Input: part model. Units: mm. Frame: model coordinates. Face numbers are marked on the shaded views. A direction names the side the tool comes from. Coordinates: 2 decimals unless noted, no trailing zeros. Loops run counter-clockwise (first coordinate to the right, second up) from the corner with the lowest first, then second, coordinate; pieces in that order, holes last. Notation, with made-up numbers: (0.5, 70) -> (35.5, 70) arc R24 cw to (35.5, 98) -> close; hole circle Ø9 at (23.25, 32.5). An arc over 180 degrees is marked (long way). Put each result on its own line as item: value. Start each with the question number.
1) Material intervals for L1, parallel to X at y = 1.75, z = -7.25; L2, parallel to Z at x = 7.62, y = 2 (3 decimals); L3, parallel to X at y = 3.25, z = 0.25, sorted ascending.
2) Cut plane B-B (z = -7). Return the cut outline in (x, y), plus the area to 3 significant figures.
3) Set-up query: the marked faces 4, 5, 6, 7 and 8. Return all of +Z, -Z, +X, -X, +Y, -Y with unobstructed straight access to the full face (end or side cutting, diameter ignored); none if empty.
4) Contact query for flat-ended pins moving along their axis: P1, Ø10, axis at x = 3, z = -1.5, coming from the -Y side; P2, Ø1.5, axis at x = 3, z = 2.5, coming from the +Y side; P3, Ø4, axis at x = 0.5, y = -3.5, coming from the -Z side. Output: stop coordinate, or through.
5) Cut plane C-C (x = 4). Return the cut outline in (y, z).
6) Pull-direction query (X, two-part tool) for the marked faces 1, 2 and 3; classes: pulls with the +X half, pulls with the -X half, needs draft (parallel to the pull), parting line crosses it, or undercut.
7) Cut plane D-D (y = -6.75). Return the cut outline in (x, z), plus the area to 3 significant figures.
8) Cut plane A-A (x = 7.62). Return the cut outline in (y, z) (3 decimals).
from build123d import *

# Parameters (mm, degrees)
ESQUISSE1_W        = 20.32
ESQUISSE1_H        = 20.32
BOSS_EXTRU_1_DEPTH = 2.7
D_GAGEMENT_M2_51_D = 2.9
ESQUISSE7_W        = 2
ESQUISSE7_H        = 2.3
ESQUISSE7_W_2      = 1.6
ESQUISSE7_H_2      = 3.2
BOSS_EXTRU_3_DEPTH = 1.1
ESQUISSE3_W        = 18.3
ESQUISSE3_H        = 2.4
BOSS_EXTRU_2_DEPTH = 8.5
CONG_1_R           = 2


with BuildPart() as part:
    # Esquisse1 → Boss.-Extru.1 (new body)
    with BuildSketch(Plane(origin=(0, 0, 0), x_dir=(1, 0, 0), z_dir=(0, 1, 0))):
        Rectangle(ESQUISSE1_W, ESQUISSE1_H)
    extrude(amount=BOSS_EXTRU_1_DEPTH)

    # Dégagement M2.51 (through all)
    with Locations(Plane(origin=(0, 2.7, 0), x_dir=(1, 0, 0), z_dir=(0, 1, 0))):
        with Locations((-7.62, 7.835000674), (7.62, 7.835000674)):
            Hole(D_GAGEMENT_M2_51_D / 2)

    # Esquisse7 → Boss.-Extru.3 (add)
    with BuildSketch(Plane(origin=(0, 2.7, 0), x_dir=(1, 0, 0), z_dir=(0, 1, 0))):
        with Locations((0.254, -0.254)):
            Rectangle(ESQUISSE7_W, ESQUISSE7_H)
        with Locations((-3.048, -0.034)):
            Rectangle(ESQUISSE7_W_2, ESQUISSE7_H_2)
    extrude(amount=BOSS_EXTRU_3_DEPTH)

    # Esquisse3 → Boss.-Extru.2 (add)
    with BuildSketch(Plane(origin=(0, 0, 0), x_dir=(1, 0, 0), z_dir=(0, 1, 0))):
        with Locations((0, -8.636)):
            Rectangle(ESQUISSE3_W, ESQUISSE3_H)
    extrude(amount=-BOSS_EXTRU_2_DEPTH)

    # Congé1
    cong_1_edges = [part.edges().sort_by_distance(p)[0] for p in [
        (-10.16, 1.35, -10.16),
        (10.16, 1.35, -10.16),
        (10.16, 1.35, 10.16),
        (-10.16, 1.35, 10.16),
    ]]
    fillet(cong_1_edges, radius=CONG_1_R)


solid = part.part
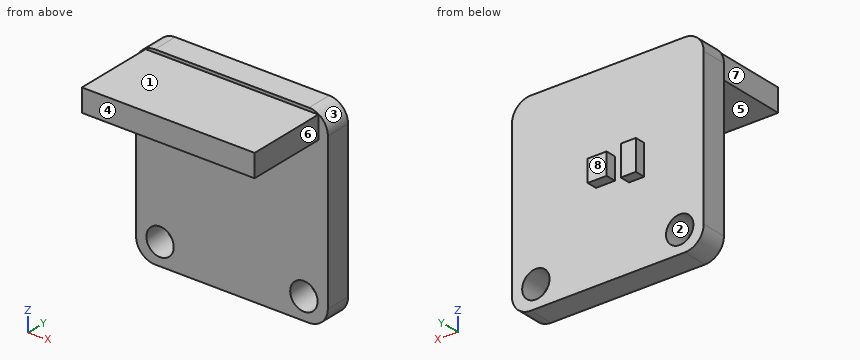
Results found:
1. L1: x = -10.16 to -8.95, -6.29 to 6.29, 8.95 to 10.16
1. L2: z = -10.16 to -9.285, -6.385 to 10.16
1. L3: x = -3.85 to -2.25, -0.75 to 1.25
2. outline: (-10.16, 0) -> (-8.81, 0) -> (-8.81, 2.7) -> (-10.16, 2.7) -> close; (-6.43, 0) -> (6.43, 0) -> (6.43, 2.7) -> (-6.43, 2.7) -> close; (8.81, 0) -> (10.16, 0) -> (10.16, 2.7) -> (8.81, 2.7) -> close
2. area: 42.1 mm2
3. face 4: +Z, -Z, +X, -X, -Y
3. face 5: -Z, +X, -X, -Y
3. face 6: +Z, -Z, +X, -Y
3. face 7: +Z, -Z, -X, -Y
3. face 8: +Z, -Z, +X, -X, +Y
4. P1: stops at y = 0
4. P2: stops at y = 2.7
4. P3: stops at z = 7.44
5. outline: (-8.5, 7.44) -> (0, 7.44) -> (0, -10.16) -> (2.7, -10.16) -> (2.7, 10.16) -> (0, 10.16) -> (0, 9.84) -> (-8.5, 9.84) -> close
6. face 1: needs draft
6. face 2: undercut
6. face 3: pulls with the +X half
7. outline: (-9.15, 7.44) -> (9.15, 7.44) -> (9.15, 9.84) -> (-9.15, 9.84) -> close
7. area: 43.9 mm2
8. outline: (-8.5, 7.436) -> (0, 7.436) -> (0, -6.385) -> (2.7, -6.385) -> (2.7, 10.16) -> (0, 10.16) -> (0, 9.836) -> (-8.5, 9.836) -> close; (0, -10.16) -> (2.7, -10.16) -> (2.7, -9.285) -> (0, -9.285) -> close
